Read the model definition and answer for the solid it produces. Units are mm, in the model's axes. Face numbers are marked on the shaded views. A direction names the side the tool comes from. Round coordinates to 2 decimals unless told otherwise and drop trailing zeros. Order: outer loops, then holes, each group sorted by start corner. A loop starts at its lowest first (then second) coordinate and runs counter-clockwise, first axis right, second up. Notation, with made-up numbers: (42, -12.5) - (60, -12.5) arc R13 ccw to (60, 0.5) - close; hole circle Ø2 at (58, 59). An arc over 180 degrees is marked (long way). One line per question, with ' | ' between items. Start each with the question number.
1) The mould has two halves that part along Y. Classify the marked faces 1, 2 and 3: pulls with the +Y half, pulls with the -Y half, needs draft (parallel to the pull), parting line crosses it, or undercut.
2) Flat-ended cylindrical pins translate along their axes: pin 1 (3 mm diameter, centred on x = 4.5, y = -3, fed in from +Z); pin 2 (1.5 mm diameter, centred on x = 9, z = 0.5, fed in from -Y) (3 decimals); pin 3 (1 mm diameter, centred on x = 8, y = 0, fed in from +Z) (3 decimals); pin 4 (2 mm diameter, centred on x = 12.5, y = 4.5, fed in from -Z). Find the tip coordinate at first contact, or state that the pin passes through.
3) Straight lines are drawn through the part: line 1 (Y direction, x = 10.5, z = 0) (3 decimals); line 2 (X direction, y = 5.25, z = 0.25); line 3 (Y direction, x = -1.25, z = 4.5). For each, find the intervals that lie inside material, in ascending order. Write a range as from..to.
4) For the marked faces 4, 5 and 6, determine the directions among +Z, -Z, +X, -X, +Y, -Y from which every point of the face is accessible in a straight line to the end or side of a thin tool.
5) The part is cut by section A-A, the plane x = 16. Give the vertices of the cut face in (y, z) (3 decimals).
Autodesk Inventor part; units mm, degrees
ref_plane "Work Plane1" through (29, 0, 0) normal (0, -1, 0) x (1, 0, 0)
ref_plane "YZ Plane" through (0, 0, 0) normal (1, 0, 0) x (0, 1, 0)
ref_plane "XZ Plane" through (0, 0, 0) normal (0, 1, 0) x (-1, 0, 0)
sketch "Sketch1" plane through (0, 0, 0) normal (0, 0, 1) x (1, 0, 0)
  line L0 (0.1778, 0) -> (19.05, 0)
  line L1 (19.05, 0) -> (19.05, 3.175)
  line L2 (19.05, 3.175) -> (2.5402, 3.175)
  line L3 (2.5402, 3.175) -> (0.0001, 3.175)
  line L4 (0.0001, 3.175) -> (0, 3.175)
  line L5 (0, 3.175) -> (0, 5.5499)
  line L6 (0, 5.5499) -> (-3.3528, 5.5499)
  line L7 (-3.3528, 5.5499) -> (-3.3528, 2.2877)
  line L8 (-3.3528, 2.2877) -> (-1.143, 2.2877)
  line L9 (-1.143, 2.2877) -> (0.1778, 0)
  line L10 (-7.8334, 0) -> (23.5306, 0)
  line L11 (0, -1.11) -> (0, 6.6599)
  line L12 (2.5402, 3.175) -> (0, 3.175) construction
  dimension "d1" = 16.5098
  dimension "d2" = 2.5401
  dimension "d3" = 3.3528
  dimension "d4" = 2.2098
  dimension "d5" = 60
  dimension "d6" = 6.35
  dimension "d7" = 6.35
  dimension "d8" = 4.5754
  dimension "d9" = 11.0998
  dimension "d26" = 19.05
revolve "Body" add sketch "Sketch1" angle 360 about axis through (0.1778, 0, 0) along (1, 0, 0) contours L9 L11 L3 L2 L1 L0 | L9 L8 L7 L6 L5 L11
sketch "Sketch2" plane through (-3.3528, 0, 0) normal (-1, 0, 0) x (0, 0, 1)
  circle A0 centre (0, 0) radius 2.2877
  line L0 (0, -7.7699) -> (0, 7.7699)
  line L1 (-7.7699, 0) -> (7.7699, 0)
  line L2 (2.2877, 0) -> (1.1438, -1.9812)
  line L3 (1.1438, -1.9812) -> (-1.1438, -1.9812)
  line L4 (-1.1438, -1.9812) -> (-2.2877, 0)
  line L5 (-2.2877, 0) -> (-1.1438, 1.9812)
  line L6 (-1.1438, 1.9812) -> (1.1438, 1.9812)
  line L7 (1.1438, 1.9812) -> (2.2877, 0)
extrude "Slot" add sketch "Sketch2" against normal up to next contours L7 A0 | A0 L2 | L6 L0 A0 | A0 L0 L3 | L0 L6 A0 | A0 L3 L0 | L4 A0 | A0 L5
fillet "Fillet1" radius 2.9718 1 edges at (-3.3528, -5.5499, 0)
thread "Thread"
chamfer "Chamfer1" distance 0.779 distance2 0.779 1 edges at (19.05, -3.175, 0) measured on face at (19.05, 0.0983, -0.8099)
ref_plane "Work Plane1" through (29, 0, 0) normal (0, -1, 0) x (1, 0, 0)
fillet "Fillet2" radius 0.1 1 edges at (0.0001, -3.175, 0)
equation "\"d30\" = R"
equation "\"d17\" = RR"
equation "\"d13\" = GEL"
equation "\"d15\" = -0.5 * SPD + 0.5 * GD"
equation "\"d16\" = GUL"
equation "\"d1\" = GEL"
equation "\"d3\" = KOH"
equation "\"d4\" = INTI"
equation "\"d6\" = GD"
equation "\"d7\" = BDM"
equation "\"d8\" = 1.1547 * SW"
equation "\"d9\" = KOD"
equation "\"d26\" = NLG"
equation "\"GD\" = NND"
equation "\"NLG\" = 19.05"
equation "\"GEL\" = 16.5098"
equation "\"KOD\" = 11.0998"
equation "\"KOH\" = 3.3528"
equation "\"INTI\" = 2.2098"
equation "\"GAL\" = 2.54"
equation "\"GUL\" = 0.77902"
equation "\"BDM\" = NND"
equation "\"SW\" = 3.9624"
equation "\"RR\" = 2.9718"
equation "\"SPD\" = 4.79196"
equation "\"R\" = 0.1"
equation "\"TOA\" = 30deg"
equation "\"GD1\" = SPD"
equation "\"THREADDIA\" = 6.35"
equation "\"KOH1\" = 0.7874"
equation "\"NND\" = 6.35"
equation "\"E0\" = 4.57657"
properties part number "ANSI B18.3 - 1/4 - 20 x 3/4" material "Steel, Mild"
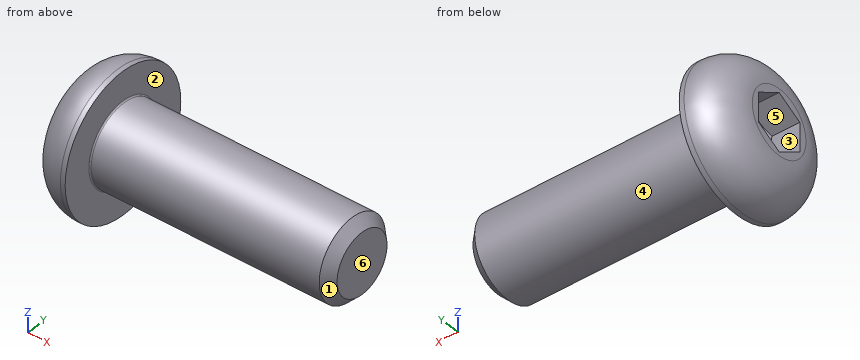
Values:
1) face 1: parting line crosses it | face 2: needs draft | face 3: undercut
2) pin 1: stops at z = 2.8 | pin 2: stops at y = -3.175 | pin 3: stops at z = 3.175 | pin 4: passes through
3) line 1: y = -3.175..3.175 | line 2: x = -1.67..0 | line 3: y = -3.02..3.02
4) face 4: +X | face 5: -X | face 6: +Z, -Z, +X, +Y, -Y
5) outline: circle Ø6.35 at (0, 0)
